from build123d import *

# Parameters (mm, degrees)
BOSS_EXTRUDE4_DEPTH  = 1.5
SKETCH5_W            = 155
SKETCH5_H            = 54
BOSS_EXTRUDE5_DEPTH  = 1.5
SKETCH8_W            = 1.5
SKETCH8_H            = 330
BOSS_EXTRUDE14_DEPTH = 4
SKETCH7_W            = 155
SKETCH7_H            = 54
BOSS_EXTRUDE18_DEPTH = 1.5
SKETCH9_W            = 333
SKETCH9_H            = 54
BOSS_EXTRUDE19_DEPTH = 1.5
SKETCH10_R           = 2.1
CUT_EXTRUDE1_DEPTH   = 10
CUT_EXTRUDE2_START   = -10
SKETCH17_R           = 2.1
CUT_EXTRUDE2_DEPTH   = 10
SKETCH16_R           = 2.1
CUT_EXTRUDE3_DEPTH   = 10
CUT_EXTRUDE4_START   = -10
SKETCH11_R           = 2.1
CUT_EXTRUDE4_DEPTH   = 10
SKETCH12_R           = 2.1
CUT_EXTRUDE5_DEPTH   = 10
SKETCH13_R           = 2.1
CUT_EXTRUDE6_DEPTH   = 10
CUT_EXTRUDE7_START   = -10
SKETCH14_R           = 2.1
CUT_EXTRUDE7_DEPTH   = 10
CUT_EXTRUDE8_START   = -10
SKETCH15_R           = 2.1
CUT_EXTRUDE8_DEPTH   = 10
SKETCH18_W           = 40.776716255
SKETCH18_H           = 21.003646254
CUT_EXTRUDE9_DEPTH   = 10
SKETCH21_W           = 37.24685685
SKETCH21_H           = 36.694897388
CUT_EXTRUDE12_DEPTH  = 10


with BuildPart() as part:
    # Sketch4 → Boss-Extrude4 (new body)
    with BuildSketch(Plane(origin=(0, 0, 0), x_dir=(1, 0, 0), z_dir=(0, 1, 0))):
        Polygon((179.47837592, 330), (334.47837592, 330), (334.47837592, 0), (179.47837592, 0), (179.47837592, 200), (179.47837592, 265), align=None)
    extrude(amount=BOSS_EXTRUDE4_DEPTH)

    # Sketch5 → Boss-Extrude5 (add)
    with BuildSketch(Plane.XY):
        with Locations((256.97837592, -25.5)):
            Rectangle(SKETCH5_W, SKETCH5_H)
    extrude(amount=BOSS_EXTRUDE5_DEPTH)

    # Sketch8 → Boss-Extrude14 (add)
    with BuildSketch(Plane(origin=(0, 1.5, 0), x_dir=(1, 0, 0), z_dir=(0, 1, 0))):
        with Locations((333.72837592, 165)):
            Rectangle(SKETCH8_W, SKETCH8_H)
    extrude(amount=BOSS_EXTRUDE14_DEPTH)

    # Sketch7 → Boss-Extrude18 (add)
    with BuildSketch(Plane(origin=(0, 0, -330), x_dir=(-1, 0, 0), z_dir=(0, 0, -1))):
        with Locations((-256.97837592, -25.5)):
            Rectangle(SKETCH7_W, SKETCH7_H)
    extrude(amount=BOSS_EXTRUDE18_DEPTH)

    # Sketch9 → Boss-Extrude19 (add)
    with BuildSketch(Plane.ZY.offset(-179.47837592)):
        with Locations((-165, -25.5)):
            Rectangle(SKETCH9_W, SKETCH9_H)
    extrude(amount=BOSS_EXTRUDE19_DEPTH)

    # Sketch10 → Cut-Extrude1 (cut)
    with BuildSketch(Plane(origin=(0, 0, -331.5), x_dir=(-1, 0, 0), z_dir=(0, 0, -1))):
        with Locations((-209.47837592, -42.5)):
            Circle(SKETCH10_R)
    extrude(amount=-CUT_EXTRUDE1_DEPTH, mode=Mode.SUBTRACT)

    # Sketch17 → Cut-Extrude2 (cut)
    with BuildSketch(Plane.XY.offset(1.5).offset(CUT_EXTRUDE2_START)):
        with Locations(Location((209.47837592, -42.5, 0), (0, 0, 180))):
            Circle(SKETCH17_R)
    extrude(amount=CUT_EXTRUDE2_DEPTH, mode=Mode.SUBTRACT)

    # Sketch16 → Cut-Extrude3 (cut)
    with BuildSketch(Plane.XY.offset(1.5)):
        with Locations((189.47837592, -42.5)):
            Circle(SKETCH16_R)
    extrude(amount=-CUT_EXTRUDE3_DEPTH, mode=Mode.SUBTRACT)

    # Sketch11 → Cut-Extrude4 (cut)
    with BuildSketch(Plane(origin=(0, 0, -331.5), x_dir=(-1, 0, 0), z_dir=(0, 0, -1)).offset(CUT_EXTRUDE4_START)):
        with Locations(Location((-189.47837592, -42.5, 0), (0, 0, 180))):
            Circle(SKETCH11_R)
    extrude(amount=CUT_EXTRUDE4_DEPTH, mode=Mode.SUBTRACT)

    # Sketch12 → Cut-Extrude5 (cut)
    with BuildSketch(Plane(origin=(0, 0, -331.5), x_dir=(-1, 0, 0), z_dir=(0, 0, -1))):
        with Locations((-189.47837592, -22.5)):
            Circle(SKETCH12_R)
    extrude(amount=-CUT_EXTRUDE5_DEPTH, mode=Mode.SUBTRACT)

    # Sketch13 → Cut-Extrude6 (cut)
    with BuildSketch(Plane(origin=(0, 0, -331.5), x_dir=(-1, 0, 0), z_dir=(0, 0, -1))):
        with Locations((-209.47837592, -22.5)):
            Circle(SKETCH13_R)
    extrude(amount=-CUT_EXTRUDE6_DEPTH, mode=Mode.SUBTRACT)

    # Sketch14 → Cut-Extrude7 (cut)
    with BuildSketch(Plane.XY.offset(1.5).offset(CUT_EXTRUDE7_START)):
        with Locations(Location((189.47837592, -22.5, 0), (0, 0, 180))):
            Circle(SKETCH14_R)
    extrude(amount=CUT_EXTRUDE7_DEPTH, mode=Mode.SUBTRACT)

    # Sketch15 → Cut-Extrude8 (cut)
    with BuildSketch(Plane.XY.offset(1.5).offset(CUT_EXTRUDE8_START)):
        with Locations(Location((209.47837592, -22.5, 0), (0, 0, 180))):
            Circle(SKETCH15_R)
    extrude(amount=CUT_EXTRUDE8_DEPTH, mode=Mode.SUBTRACT)

    # Sketch18 → Cut-Extrude9 (cut)
    with BuildSketch(Plane(origin=(0, 1.5, 0), x_dir=(1, 0, 0), z_dir=(0, 1, 0))):
        with Locations((199.375823154, 209.882956498)):
            Rectangle(SKETCH18_W, SKETCH18_H)
    extrude(amount=-CUT_EXTRUDE9_DEPTH, mode=Mode.SUBTRACT)

    # Sketch21 → Cut-Extrude12 (cut)
    with BuildSketch(Plane(origin=(0, 1.5, 0), x_dir=(1, 0, 0), z_dir=(0, 1, 0))):
        with Locations((238.101804345, 271.652551306)):
            Rectangle(SKETCH21_W, SKETCH21_H)
    extrude(amount=-CUT_EXTRUDE12_DEPTH, mode=Mode.SUBTRACT)


solid = part.part
Part model, mm, in its own coordinate system. A direction names the side the tool comes from. Coordinates: 2 decimals unless noted, no trailing zeros. Order: outer loops, then holes, each group sorted by start corner. A loop starts at its lowest first (then second) coordinate and runs counter-clockwise, first axis right, second up. Notation, with made-up numbers: (65, 13.25) - (116, 13.25) arc R18 ccw to (116, 43.25) - close; hole circle Ø1 at (56, -38.5). An arc over 180 degrees is marked (long way). Use CSV: the item, a comma, the result in double quotes.
Item 1: Saw through at B-B on z = -282.5. Give the cut face in (x, y), and give its area (3 significant figures).
Solved:
outline,"(177.98, -52.5) - (179.48, -52.5) - (179.48, 0) - (219.48, 0) - (219.48, 1.5) - (177.98, 1.5) - close; (256.73, 0) - (334.48, 0) - (334.48, 5.5) - (332.98, 5.5) - (332.98, 1.5) - (256.73, 1.5) - close"
area,"264 mm²"
Item 2: Saw through at D-D on x = 293. Give the cut face in (y, z), and give its area (3 significant figures).
Solved:
outline,"(-52.5, -331.5) - (1.5, -331.5) - (1.5, 1.5) - (-52.5, 1.5) - (-52.5, 0) - (0, 0) - (0, -330) - (-52.5, -330) - close"
area,"657 mm²"
Item 3: Drop flat-ended pins along their axis: P1, Ø2, axis at y = -31.5, z = -279.5, coming from the +X side; P2, Ø3, axis at x = 318, z = -88.5, coming from the -Y side; P3, Ø5, axis at x = 274.5, z = -172, coming from the +Y side. Give the stop position or say it passes through.
Solved:
P1,"stops at x = 179.48"
P2,"stops at y = 0"
P3,"stops at y = 1.5"
Item 4: Mould opens along Z. For faces 1 (the face through (177.978, -25, -167)), 2 (the face through (257, -26, 1.5)), 3 (the face through (256, -26, 0)) say: +Z half, -Z half, draft (parallel to the pull), parting line (faces both ways), or undercut.
Solved:
face 1,"draft"
face 2,"+Z half"
face 3,"undercut"
Item 5: Saw through at A-A on x = 247. Give the cut face in (y, z), and give its area (3 significant figures).
Solved:
outline,"(-52.5, -331.5) - (1.5, -331.5) - (1.5, -290) - (0, -290) - (0, -330) - (-52.5, -330) - close; (-52.5, 0) - (0, 0) - (0, -253.31) - (1.5, -253.31) - (1.5, 1.5) - (-52.5, 1.5) - close"
area,"602 mm²"
Item 6: Saw through at C-C on y = -14.5. Give the cut face in (x, z), and give its area (4 significant figures).
Solved:
outline,"(177.98, -331.5) - (334.48, -331.5) - (334.48, -330) - (179.48, -330) - (179.48, 0) - (334.48, 0) - (334.48, 1.5) - (177.98, 1.5) - close"
area,"964.5 mm²"
Item 7: Probe probe 1 along X at (y, z) = (-22.5, 0.7); probe 2 along Z at (x, y) = (247, -21); probe 3 along Y at (x, z) = (206, -61). List the from-to ranges inside material, lowest first.
Solved:
probe 1,"x = 177.98 to 187.38, 191.58 to 207.38, 211.58 to 334.48"
probe 2,"z = -331.5 to -330, 0 to 1.5"
probe 3,"y = 0 to 1.5"
Item 8: 3-axis set-ups, long thin cutter, end or side, ignore diameter. For faces 4 (the face through (179.478, -26, -167)), 5 (the face through (257, -26, -331.5)): which of +Z, -Z, +X, -X, +Y, -Y reach the whole face in a straight line?
Solved:
face 4,"+X, -Y"
face 5,"-Z, +X, -X, +Y, -Y"
